Autodesk Inventor part; units mm, degrees
ref_plane "YZ Plane" through (0, 0, 0) normal (1, 0, 0) x (0, 1, 0)
ref_plane "XZ Plane" through (0, 0, 0) normal (0, 1, 0) x (-1, 0, 0)
ref_plane "XY Plane" through (0, 0, 0) normal (0, 0, 1) x (1, 0, 0)
sketch "Sketch11" plane through (0, 0, 0) normal (0, 1, 0) x (-1, 0, 0)
  arc A0 (2.6519, 1.7) -> (2.6519, -1.7) centre (0, 0) ccw
  line L0 (2.6519, 1.7) -> (2.6519, -1.7)
  line L1 (12.5, 12.5) -> (-12.5, 12.5)
  line L2 (-12.5, 12.5) -> (-12.5, -12.5)
  line L3 (-12.5, -12.5) -> (12.5, -12.5)
  line L4 (12.5, -12.5) -> (12.5, 12.5)
  line L5 (12.5, 12.5) -> (-12.5, -12.5) construction
  line L6 (-12.5, 12.5) -> (12.5, -12.5) construction
  dimension "d45" = 6.3
  dimension "d46" = 3.4
  dimension "d47" = 25
  dimension "d48" = 25
extrude "Extrusion8" add sketch "Sketch11" along normal blind 40
sketch "Sketch12" plane through (0, 40, 0) normal (0, 1, 0) x (1, 0, 0)
  line L0 (0, -7.3612) -> (6.375, -3.6806)
  line L1 (6.375, -3.6806) -> (6.375, 3.6806)
  line L2 (6.375, 3.6806) -> (0, 7.3612)
  line L3 (0, 7.3612) -> (-6.375, 3.6806)
  line L4 (-6.375, 3.6806) -> (-6.375, -3.6806)
  line L5 (-6.375, -3.6806) -> (0, -7.3612)
  line L6 (0, -7.3612) -> (0, 0)
  line L7 (0, 0) -> (0, 7.3612)
  point P0 (3.1875, -5.5209)
  dimension "d52" = 120
  dimension "d54" = 12.75
extrude "Extrusion9" cut sketch "Sketch12" against normal blind 20
sketch "Sketch13" plane through (0, 40, 0) normal (0, 1, 0) x (1, 0, 0)
  line L0 (-7.9375, -3) -> (-10.9375, -3)
  line L1 (-10.9375, -3) -> (-10.9375, 3)
  line L2 (-10.9375, 3) -> (-7.9375, 3)
  line L3 (-7.9375, 3) -> (-7.9375, -3)
  line L4 (-7.9375, -3) -> (-10.9375, 3) construction
  line L5 (-10.9375, -3) -> (-7.9375, 3) construction
  line L6 (-12.5, 12.5) -> (-12.5, -12.5)
  point P0 (0, 0)
  point P1 (-9.4375, 0)
  dimension "d57" = 3
  dimension "d58" = 6
  dimension "d59" = 3.0625
extrude "Extrusion10" cut sketch "Sketch13" against normal blind 10
sketch "Sketch14" plane through (-7.9375, 40, -3) normal (-1, 0, 0) x (0, 0, 1)
  circle A0 centre (3, -5) radius 1.5
  line L0 (6, 0) -> (6, -10)
  line L1 (6, -10) -> (0, -10)
  point P0 (3, -40)
  dimension "d62" = 3
  dimension "d63" = 3
  dimension "d64" = 5
extrude "Extrusion11" cut sketch "Sketch14" along normal mid plane 10
sketch "Sketch15" plane through (0, 0, 0) normal (0, -1, 0) x (1, 0, 0)
  line L0 (-10.937, -3) -> (-7.937, -3)
  line L1 (-7.937, -3) -> (-7.937, 3)
  line L2 (-7.937, 3) -> (-10.937, 3)
  line L3 (-10.937, 3) -> (-10.937, -3)
  line L4 (-12.5, -12.5) -> (-12.5, 12.5)
  point P0 (0, 0)
  point P1 (-9.437, 3)
  dimension "d67" = 3
  dimension "d68" = 6
  dimension "d69" = 4.563
  dimension "d70" = 3
extrude "Extrusion12" cut sketch "Sketch15" against normal blind 10
sketch "Sketch16" plane through (-7.937, 0, -3) normal (-1, 0, 0) x (0, 0, 1)
  circle A0 centre (3, 5) radius 1.5
  line L0 (6, 0) -> (6, 10)
  line L1 (-9.5, 0) -> (15.5, 0)
  point P0 (3, 0)
  dimension "d73" = 3
  dimension "d74" = 3
  dimension "d75" = 5
extrude "Extrusion13" cut sketch "Sketch16" along normal blind 10 and the other way blind 6
fillet "Fillet1" radius 8 4 edges at (12.5, 20, -12.5) (12.5, 20, 12.5) (-12.5, 20, -12.5) (-12.5, 20, 12.5)
properties part number "collar"
The listing builds one solid part. Answer for the finished solid, in the listing's coordinates (mm). A direction names the side the tool comes from. Give positions to 0.01 mm unless a question says otherwise; leave off trailing zeros. Order: outer loops, then holes, each group sorted by start corner. A loop starts at its lowest first (then second) coordinate and runs counter-clockwise, first axis right, second up.
1) Determine the mould class of faces 1 (the face through (-10.219, 20.28, 10.094)), 2 (the face through (-11.708, 36.464, -0.325)), 3 (the face through (-7.938, 36.2, 1.3)), 4 (the face through (-12.5, 20, 0)) for opening direction Z: pulls with the +Z half, pulls with the -Z half, needs draft (parallel to the pull), parting line crosses it, or undercut.
Reported:
face 1: pulls with the +Z half
face 2: undercut
face 3: undercut
face 4: needs draft
2) Consider line 1 along X through (y, z) = (38.5, -0.75) (1 decimal); line 2 along Y through (x, z) = (-11.35, 0); line 3 along Z through (x, y) = (0, 12.25). Determine where each line is inside the solid, lowest interval first.
Reported:
line 1: x = -12.5 to -10.9, -7.9 to -6.4, 6.4 to 12.5
line 2: y = 0 to 3.5, 6.5 to 33.5, 36.5 to 40
line 3: z = -12.5 to -3.15, 3.15 to 12.5
3) Find section A-A on y = 26.5. Write down the section's boundary in (x, z) (3 decimals), then the cut area to 3 significant figures.
Reported:
outline: (-12.5, -4.5) arc R8 ccw to (-4.5, -12.5) - (4.5, -12.5) arc R8 ccw to (12.5, -4.5) - (12.5, 4.5) arc R8 ccw to (4.5, 12.5) - (-4.5, 12.5) arc R8 ccw to (-12.5, 4.5) - close; hole (-6.375, -3.681) - (0, -7.361) - (6.375, -3.681) - (6.375, 3.681) - (0, 7.361) - (-6.375, 3.681) - close
area: 429 mm2
4) Find section C-C on x = -3.25. Write down the section's boundary in (y, z).
Reported:
outline: (0, -12.5) - (40, -12.5) - (40, -5.48) - (20, -5.48) - (20, 5.48) - (40, 5.48) - (40, 12.5) - (0, 12.5) - close; hole circle Ø3 at (5, 0)
5) For faces 5 (the face through (-5.33, 5.07, -1.5)), 6 (the face through (-3, 20, 0)), 7 (the face through (-7.937, 3.8, 1.3)), determine the directions among +Z, -Z, +X, -X, +Y, -Y from which every point of the face is accessible in a straight line to the end or side of a thin tool.
Reported:
face 5: -X
face 6: +Y
face 7: -Y
6) Find section D-D on z = 0. Give the number of separate pieces and of enclosed holes in the cut face, then the cut area to 3 significant figures.
Reported:
separate pieces: 6
enclosed holes: 0
area: 539 mm2
7) Given P1, Ø0.9, axis at x = -10, y = 5, coming from the -Z side; P2, Ø4, axis at y = 35.5, z = -7.5, coming from the +X side; P3, Ø1.8, axis at y = 36, z = 0.5, coming from the -X side; P4, Ø2.5, axis at x = -9.5, y = 34, coming from the -Z side, each flat-ended and moving along its own axis, determine where each tip first touches the part or whether it passes through.
Reported:
P1: stops at z = -10.7
P2: stops at x = 12.44
P3: stops at x = -12.5
P4: stops at z = -11.57
8) Find section B-B on y = 35. Write down the section's boundary in (x, z) (1 decimal).
Reported:
outline: (-12.5, -4.5) arc R8 ccw to (-4.5, -12.5) - (4.5, -12.5) arc R8 ccw to (12.5, -4.5) - (12.5, 4.5) arc R8 ccw to (4.5, 12.5) - (-4.5, 12.5) arc R8 ccw to (-12.5, 4.5) - (-12.5, 1.5) - (-10.9, 1.5) - (-10.9, 3) - (-7.9, 3) - (-7.9, 1.5) - (-6.4, 1.5) - (-6.4, 3.7) - (0, 7.4) - (6.4, 3.7) - (6.4, -3.7) - (0, -7.4) - (-6.4, -3.7) - (-6.4, -1.5) - (-7.9, -1.5) - (-7.9, -3) - (-10.9, -3) - (-10.9, -1.5) - (-12.5, -1.5) - close
